Source: CAD feature listing. Evaluate the final solid. Frame: model axes, mm. A direction names the side the tool comes from. Give positions to 0.01 mm unless a question says otherwise; leave off trailing zeros. Loops run counter-clockwise (first coordinate to the right, second up) from the corner with the lowest first, then second, coordinate; pieces in that order, holes last. Notation, with made-up numbers: (21, -22) -> (69, -22) arc R10 cw to (69, -6) -> close; hole circle Ø4 at (7, 25). An arc over 180 degrees is marked (long way). Return JSON: item names as keys, results as strings. Group by question number.
```python
from build123d import *

# Parameters (mm, degrees)
SKETCH1_R               = 5
BOSS_EXTRUDE1_DEPTH     = 36
SKETCH2_R               = 9
BOSS_EXTRUDE2_DEPTH     = 3
CUT_EXTRUDE1_DEPTH      = 39.183766184
CUT_EXTRUDE1_DEPTH_BACK = 39.183766184
SKETCH3_R               = 1.5


with BuildPart() as part:
    # Sketch1 → Boss-Extrude1 (new body)
    with BuildSketch(Plane.XY):
        Circle(SKETCH1_R)
    extrude(amount=BOSS_EXTRUDE1_DEPTH)

    # Sketch2 → Boss-Extrude2 (add)
    with BuildSketch(Plane.XY):
        Circle(SKETCH2_R)
    extrude(amount=-BOSS_EXTRUDE2_DEPTH)

    # Sketch3 → Cut-Extrude1 (cut, two sides: drawn at the far end of the back side and taken through both)
    with BuildSketch(Plane(origin=(0, 0, 0), x_dir=(0, 0, -1), z_dir=(1, 0, 0)).offset(-CUT_EXTRUDE1_DEPTH_BACK)):
        with Locations(Location((-33, 0, 0), (0, 0, 179.999999999))):
            Circle(SKETCH3_R)
    extrude(amount=CUT_EXTRUDE1_DEPTH + CUT_EXTRUDE1_DEPTH_BACK, mode=Mode.SUBTRACT)


solid = part.part
```
1) Cut plane B-B on y = 0. Return loops of the section in (x, z).
2) Contact query for flat-ended pins moving along their axis: P1, Ø3, axis at x = 3.5, z = 23.5, coming from the +Y side; P2, Ø5, axis at y = 3, z = 7, coming from the -X side; P3, Ø6, axis at y = -1.5, z = 6, coming from the +X side. Output: stop coordinate, or through.
3) Cut plane C-C on y = -2.5. Return loops of the section in (x, z), then the cut area to 3 significant figures.
4) Cut plane D-D on z = 13.5. Return loops of the section in (x, y).
5) Cut plane A-A on x = 0. Return loops of the section in (y, z).
6) Material intervals for line 1 (Y direction, x = -1.25, z = 33); line 2 (Z direction, x = 7.25, y = -4.75); line 3 (Y direction, x = -3.5, z = 34), sorted ascending.
7) Mould query, pull axis Y, two halves, no side actions, for faces 3 (the face through (4, -4, 0)), 4 (the face through (-0.07, -0.45, 34.43)), 5 (the face through (-1.172, 8.923, -1.479)). Classes: released by +Y, released by -Y, zero draft, split by the parting line, or undercut.
8) Reachability of faces 1 (the face through (0, 0, 36)), 2 (the face through (4.619, -1.915, 17.748)) from +Z, -Z, +X, -X, +Y, -Y: full face, straight path, thin tool, end or side. Return the list, or none.
Calculated:
{
 "1": {"outline": "(-9, -3) -> (9, -3) -> (9, 0) -> (5, 0) -> (5, 31.5) -> (-5, 31.5) -> (-5, 0) -> (-9, 0) -> close; (-5, 34.5) -> (5, 34.5) -> (5, 36) -> (-5, 36) -> close"},
 "2": {"P1": "y = 4.58", "P2": "x = -4.97", "P3": "x = 5"},
 "3": {"outline": "(-8.65, -3) -> (8.65, -3) -> (8.65, 0) -> (4.33, 0) -> (4.33, 36) -> (-4.33, 36) -> (-4.33, 0) -> (-8.65, 0) -> close", "area": "364 mm2"},
 "4": {"outline": "circle Ø10 at (0, 0)"},
 "5": {"outline": "(-9, -3) -> (9, -3) -> (9, 0) -> (5, 0) -> (5, 36) -> (-5, 36) -> (-5, 0) -> (-9, 0) -> close; hole circle Ø3 at (0, 33)"},
 "6": {"line 1": "-4.84 to -1.5, 1.5 to 4.84", "line 2": "-3 to 0", "line 3": "-3.57 to -1.12, 1.12 to 3.57"},
 "7": {"face 3": "zero draft", "face 4": "undercut", "face 5": "split by the parting line"},
 "8": {"face 1": "+Z, +X, -X, +Y, -Y", "face 2": "+Z"}
}
